Source: CAD feature listing. Evaluate the final solid. Frame: model axes, mm. A direction names the side the tool comes from. Give positions to 0.01 mm unless a question says otherwise; leave off trailing zeros. Loops run counter-clockwise (first coordinate to the right, second up) from the corner with the lowest first, then second, coordinate; pieces in that order, holes last.
```python
from build123d import *

# Parameters (mm, degrees)
F0_W      = 16
F0_H      = 16
F1_DEPTH  = 3
F2_R      = 2.45
F3_DEPTH  = 1.8
F4_R      = 1.800771
F5_DEPTH  = 2.5
F6_R      = 1.5
F7_DEPTH  = 25
F8_R      = 1.75
F9_DEPTH  = 1
F11_DEPTH = 1
F13_DEPTH = 1
F14_R     = 1.446207
F15_DEPTH = 25
F16_R     = 1.75
F17_DEPTH = 1
F19_DEPTH = 1


with BuildPart() as f1:
    # F0 (on Front) → F1 (new body)
    with BuildSketch(Plane.XZ):
        Rectangle(F0_W, F0_H)
    extrude(amount=F1_DEPTH)

    # F2 (on face) → F3 (join)
    with BuildSketch(Plane.XZ.offset(3)):
        with Locations((-4.2, 4.2)):
            Circle(F2_R)
        with Locations((4.2, 4.2)):
            Circle(F2_R)
        with Locations((-4.2, -4.2)):
            Circle(F2_R)
        with Locations((4.2, -4.2)):
            Circle(F2_R)
    extrude(amount=F3_DEPTH)

    # F4 (on face) → F5 (join)
    with BuildSketch(Plane.YZ.offset(8)):
        with Locations((-1.199229, 0)):
            Circle(F4_R)
    extrude(amount=F5_DEPTH)

    # F6 (on face) → F7 (join)
    with BuildSketch(Plane.YZ.offset(10.5)):
        with Locations((-1.199229, 0)):
            Circle(F6_R)
    extrude(amount=F7_DEPTH)

    # F8 (on face) → F9 (join)
    with BuildSketch(Plane.YZ.offset(35.5)):
        with Locations((-1.199229, 0)):
            Circle(F8_R)
    extrude(amount=-F9_DEPTH)

    # F10 (on face) → F11 (cut)
    with BuildSketch(Plane.YZ.offset(35.5)):
        with BuildLine():
            Line((0.477822, 0.5), (-2.87628, 0.5))
            ThreePointArc((-2.87628, 0.5), (-2.949229, 0), (-2.87628, -0.5))
            Line((-2.87628, -0.5), (0.477822, -0.5))
            ThreePointArc((0.477822, -0.5), (0.532437, -0.252647), (0.550771, 0))
            ThreePointArc((0.550771, 0), (0.532437, 0.252647), (0.477822, 0.5))
        make_face()
    extrude(amount=-F11_DEPTH, mode=Mode.SUBTRACT)

    # F12 (on face) → F13 (join)
    with BuildSketch(Plane(origin=(-8, 0, 0), x_dir=(0, -1, 0), z_dir=(-1, 0, 0))):
        with BuildLine():
            ThreePointArc((-0.59449, 0), (1.202755, -1.797245), (3, 0))
            Line((3, 0), (-0.59449, 0))
        make_face()
        with BuildLine():
            Line((-0.59449, 0), (3, 0))
            ThreePointArc((3, 0), (1.202755, 1.797245), (-0.59449, 0))
        make_face()
    extrude(amount=F13_DEPTH)

    # F14 (on face) → F15 (join)
    with BuildSketch(Plane(origin=(-9, 0, 0), x_dir=(0, -1, 0), z_dir=(-1, 0, 0))):
        with Locations((1.202755, 0)):
            Circle(F14_R)
    extrude(amount=F15_DEPTH)

    # F16 (on face) → F17 (join)
    with BuildSketch(Plane(origin=(-34, 0, 0), x_dir=(0, -1, 0), z_dir=(-1, 0, 0))):
        with Locations((1.202755, 0)):
            Circle(F16_R)
    extrude(amount=F17_DEPTH)

    # F18 (on face) → F19 (cut)
    with BuildSketch(Plane(origin=(-35, 0, 0), x_dir=(0, -1, 0), z_dir=(-1, 0, 0))):
        with BuildLine():
            Line((2.879806, 0.5), (-0.474296, 0.5))
            ThreePointArc((-0.474296, 0.5), (-0.547245, 0), (-0.474296, -0.5))
            Line((-0.474296, -0.5), (2.879806, -0.5))
            ThreePointArc((2.879806, -0.5), (2.934422, -0.252647), (2.952755, 0))
            ThreePointArc((2.952755, 0), (2.934422, 0.252647), (2.879806, 0.5))
        make_face()
    extrude(amount=-F19_DEPTH, mode=Mode.SUBTRACT)


solid = f1.part
```
(1) Section A-A, the plane x = -4.2. Return the cut outline in (y, z), then the cut area to 3 significant figures.
A:
outline: (-4.8, -6.65) - (-3, -6.65) - (-3, -8) - (0, -8) - (0, 8) - (-3, 8) - (-3, 6.65) - (-4.8, 6.65) - (-4.8, 1.75) - (-3, 1.75) - (-3, -1.75) - (-4.8, -1.75) - close
area: 65.6 mm2
(2) Section C-C, the plane x = -14.5. Return the cut outline in (y, z).
A:
outline: circle Ø2.89 at (-1.2, 0)
(3) Ray query, line 1 along X through (y, z) = (-1.75, 1.5); line 2 along Y through (x, z) = (-3, 2.5); line 3 along Y through (x, z) = (-1, -2.25). Return the intervals inside material, ascending.
A:
line 1: x = -35 to -34, -9 to 10.5, 34.5 to 35.5
line 2: y = -4.8 to 0
line 3: y = -3 to 0
(4) Reachability of faces 1 (the cylindrical face through (22.33, 0.23, 0.45)), 2 (the cylindrical face through (-6.144, -3.887, 2.709)), 3 (the cylindrical face through (-34.49, -1.17, -1.75)) from +Z, -Z, +X, -X, +Y, -Y: full face, straight path, thin tool, end or side. Return the list, or none.
A:
face 1: none
face 2: -Y
face 3: -Z, -X
(5) Mould query, pull axis Z, two halves, no side actions, for faces 4 (the cylindrical face through (35.01, -1.23, -1.75)), 5 (the flat face through (4, -4.8, -4)), 6 (the flat face through (0, -3, 0)), 7 (the cylindrical face through (9.232, 0.464, -0.69)). Classes: pulls with the +Z half, pulls with the -Z half, needs draft (parallel to the pull), parting line crosses it, or undercut.
A:
face 4: pulls with the -Z half
face 5: needs draft
face 6: undercut
face 7: parting line crosses it
(6) Section B-B, the plane z = -4.2. Return the cut outline in (x, y).
A:
outline: (-8, -3) - (-6.65, -3) - (-6.65, -4.8) - (-1.75, -4.8) - (-1.75, -3) - (1.75, -3) - (1.75, -4.8) - (6.65, -4.8) - (6.65, -3) - (8, -3) - (8, 0) - (-8, 0) - close
(7) First-contact query: pin 1 (0.8 mm diameter, centred on y = -1, z = 0, fed in from +X); pin 2 (0.8 mm diameter, centred on x = 35, y = -0.5, fed in from +Z); pin 3 (2 mm diameter, centred on y = -1.5, z = -2.5, fed in from +X); pin 4 (2.5 mm diameter, centred on y = -1, z = 5.5, fed in from -X). Flat tips, straight axial feed; report the tip coordinate or a pass-through.
A:
pin 1: stops at x = 34.5
pin 2: stops at z = 1.72
pin 3: stops at x = 35.5
pin 4: stops at x = -8
